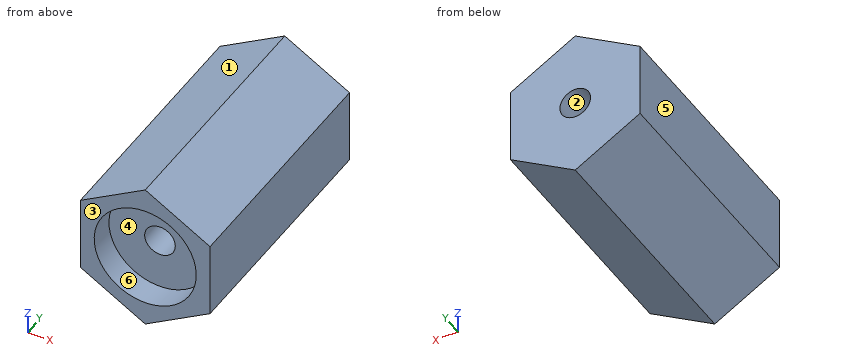
from build123d import *

# Parameters (mm, degrees)
SKETCH1_R           = 1.5
BOSS_EXTRUDE1_DEPTH = 24.0204498
SKETCH2_R           = 5
CUT_EXTRUDE1_DEPTH  = 2.54


with BuildPart() as part:
    # Sketch1 → Boss-Extrude1 (new body)
    with BuildSketch(Plane(origin=(0, 0, 0), x_dir=(1, 0, 0), z_dir=(0, 1, 0))):
        Polygon((0, 7.332348419), (-6.35, 3.666174209), (-6.35, -3.666174209), (0, -7.332348419), (6.35, -3.666174209), (6.35, 3.666174209), align=None)
        with Locations(Location((0, 0, 0), (0, 0, 270))):
            Circle(SKETCH1_R, mode=Mode.SUBTRACT)
    extrude(amount=BOSS_EXTRUDE1_DEPTH)

    # Sketch2 → Cut-Extrude1 (cut)
    with BuildSketch(Plane(origin=(0, 0, 0), x_dir=(1, 0, 0), z_dir=(0, 1, 0))):
        with Locations(Location((0, 0, 0), (0, 0, 270))):
            Circle(SKETCH2_R)
    extrude(amount=CUT_EXTRUDE1_DEPTH, mode=Mode.SUBTRACT)


solid = part.part
Source: CAD feature listing. Evaluate the final solid. Frame: model axes, mm. Face numbers are marked on the shaded views. A direction names the side the tool comes from. Give positions to 0.01 mm unless a question says otherwise; leave off trailing zeros. Loops run counter-clockwise (first coordinate to the right, second up) from the corner with the lowest first, then second, coordinate; pieces in that order, holes last. Notation, with made-up numbers: (37.5, 37) -> (84.5, 37) arc R12 ccw to (84.5, 46) -> close; hole circle Ø1 at (-8, 1.25). An arc over 180 degrees is marked (long way). Use a Markdown table: item, result. Add a question column.
1) Section query A-A, the plane z = 0. Return the cut outline in (x, y).
2) Reachability of the marked faces 5 and 6 from +Z, -Z, +X, -X, +Y, -Y: full face, straight path, thin tool, end or side. Return the list, or none.
3) Section query B-B, the plane y = 21.5. Return the cut outline in (x, z).
4) Section query C-C, the plane x = 0.75. Return the cut outline in (y, z), then the cut area to 3 significant figures.
5) Section query D-D, the plane z = 3. Return the cut outline in (x, y).
6) Pull-direction query (X, two-part tool) for the marked faces 1, 2, 3 and 4; classes: +X half, -X half, draft (parallel to the pull), parting line (faces both ways), or undercut.
7) Line query: line 1 along X through (y, z) = (1.45, 0); line 2 along X through (y, z) = (17.5, 0); line 3 along Y through (x, z) = (2.5, 4). Output: solid intervals per line, ascending. Write a range as [from, to].
8) First-contact query: pin 1 (3.5 mm diameter, centred on x = 0, z = 0, fed in from -Y). Flat tip, straight axial feed; report the tip coordinate or a pass-through.
Numbers:
| question | item | result |
|---|---|---|
| 1 | outline | (-6.35, 0) -> (-5, 0) -> (-5, 2.54) -> (-1.5, 2.54) -> (-1.5, 24.02) -> (-6.35, 24.02) -> close; (1.5, 2.54) -> (5, 2.54) -> (5, 0) -> (6.35, 0) -> (6.35, 24.02) -> (1.5, 24.02) -> close |
| 2 | face 5 | +Z, -Z, -X, +Y, -Y |
| 2 | face 6 | -Y |
| 3 | outline | (-6.35, -3.67) -> (0, -7.33) -> (6.35, -3.67) -> (6.35, 3.67) -> (0, 7.33) -> (-6.35, 3.67) -> close; hole circle Ø3 at (0, 0) |
| 4 | outline | (0, -6.9) -> (24.02, -6.9) -> (24.02, -1.3) -> (2.54, -1.3) -> (2.54, -4.94) -> (0, -4.94) -> close; (0, 4.94) -> (2.54, 4.94) -> (2.54, 1.3) -> (24.02, 1.3) -> (24.02, 6.9) -> (0, 6.9) -> close |
| 4 | area | 251 mm2 |
| 5 | outline | (-6.35, 0) -> (-4, 0) -> (-4, 2.54) -> (4, 2.54) -> (4, 0) -> (6.35, 0) -> (6.35, 24.02) -> (-6.35, 24.02) -> close |
| 6 | face 1 | -X half |
| 6 | face 2 | undercut |
| 6 | face 3 | draft |
| 6 | face 4 | undercut |
| 7 | line 1 | x = [-6.35, -5], [5, 6.35] |
| 7 | line 2 | x = [-6.35, -1.5], [1.5, 6.35] |
| 7 | line 3 | y = [2.54, 24.02] |
| 8 | pin 1 | stops at y = 2.54 |
